Job drawing, mm, ordinate dimensions from the low corner. One solid piece. A direction names the side the tool comes from. Coordinates: 2 decimals unless noted, no trailing zeros. Write each loop counter-clockwise with the first axis right and the second up, starting at its lowest first coordinate (ties: lowest second). Pieces come first, ordered by that corner, then holes.
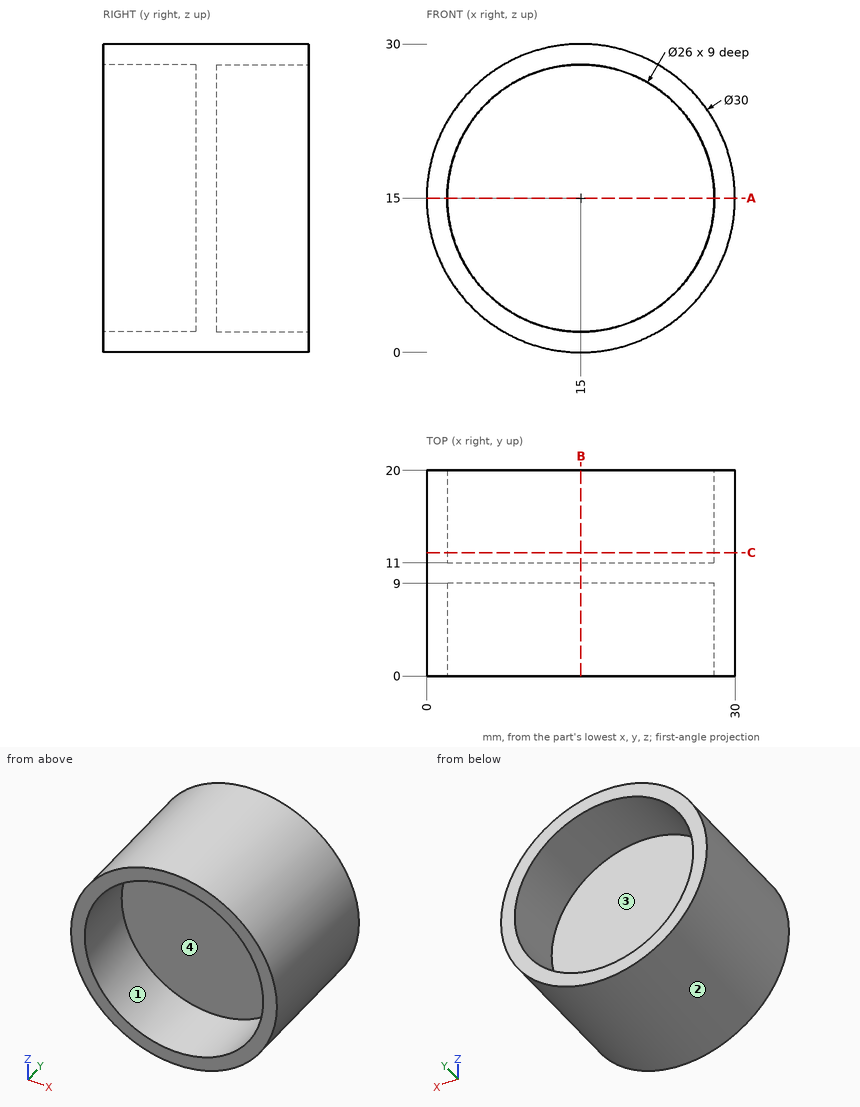
1. Mould opens along Z. For the marked faces 1 and 2 say: +Z half, -Z half, draft (parallel to the pull), parting line (faces both ways), or undercut.
Computed values:
face 1: undercut
face 2: parting line
2. Saw through at C-C on y = 12. List the corners of the cut face in (x, z), plus the area to 3 significant figures.
Computed values:
outline: circle Ø30 at (15, 15); hole circle Ø26 at (15, 15)
area: 176 mm2
3. Saw through at A-A on z = 15. List the corners of the cut face in (x, y), plus the area to 3 significant figures.
Computed values:
outline: (0, 0) - (2, 0) - (2, 9) - (28, 9) - (28, 0) - (30, 0) - (30, 20) - (28, 20) - (28, 11) - (2, 11) - (2, 20) - (0, 20) - close
area: 132 mm2
4. Saw through at B-B on x = 15. List the corners of the cut face in (y, z).
Computed values:
outline: (0, 0) - (20, 0) - (20, 2) - (11, 2) - (11, 28) - (20, 28) - (20, 30) - (0, 30) - (0, 28) - (9, 28) - (9, 2) - (0, 2) - close
5. 3-axis set-ups, long thin cutter, end or side, ignore diameter. For the marked faces 3 and 4: which of +Z, -Z, +X, -X, +Y, -Y reach the whole face in a straight line?
Computed values:
face 3: +Y
face 4: -Y
6. Flat gauge pins, fed straight in: pin 1 (12 mm diameter, centred on x = 7, y = 12, fed in from -Z); pin 2 (13 mm diameter, centred on x = 17.5, z = 10, fed in from +Y); pin 3 (13 mm diameter, centred on x = 15.5, z = 17.5, fed in from -Y). Where does each tip first touch, or does it go through?
Computed values:
pin 1: stops at z = 0.13
pin 2: stops at y = 11
pin 3: stops at y = 9
7. Probe line 1 along Z through (x, y) = (15, 17.5); line 2 along Y through (x, z) = (25, 11.5); line 3 along X through (y, z) = (12, 8.5). List the from-to ranges inside material, lowest first.
Computed values:
line 1: z = 0 to 2, 28 to 30
line 2: y = 9 to 11
line 3: x = 1.48 to 3.74, 26.26 to 28.52
